Could you check a few things on this model? Use its own coordinates, in mm. A direction names the side the tool comes from. Give positions to 0.01 mm unless a question says otherwise; leave off trailing zeros. Loops run counter-clockwise (first coordinate to the right, second up) from the corner with the lowest first, then second, coordinate; pieces in that order, holes last. Notation, with made-up numbers: M -8,-14.75 L 16,-14.75 A24 cw 16,6.25 Z; hole C -3,65.25 d4. An arc over 180 degrees is marked long. Return JSON: item names as keys, results as strings. Group by question number.
1. Please list where these lines run through material, in increasing order: line 1 (X direction, y = 329.5, z = 139.5); line 2 (Y direction, x = 30, z = -30); line 3 (Y direction, x = 3, z = 236).
2. If we mould it in two halves opening along Z, with no side actions, what happens to faces 1 (the cylindrical face through (-0.85, 342.63, 243.3)), 2 (the flat face through (13.86, 343.08, 242.65)), 3 (the flat face through (19, -3.969, -38)), 4 (the cylindrical face through (-0.98, 739.16, 387.11))? For each: +Z half, -Z half, draft (parallel to the pull), parting line (faces both ways), or undercut.
3. For faces 5 (the flat face through (-0.98, 30.1, -67.07)), 6 (the flat face through (19, -1.984, -38)), 7 (the flat face through (0, 397, 250)), 8 (the cylindrical face through (-0.978, 358.159, 168.827)), which set-ups out of +Z, -Z, +X, -X, +Y, -Y let a thin tool reach every point of the face, with its end or its side?
4. For pin 1 (2 mm diameter, centred on x = -1.5, z = 189, fed in from +Y); pin 2 (1 mm diameter, centred on x = -1, y = 765.5, fed in from -Z); pin 3 (1.6 mm diameter, centred on x = -1, y = 756, fed in from -Z); pin 4 (6.5 mm diameter, centred on y = 340.52, z = 190.1, fed in from -X), each with a flat end and sliding along its axis, tell me the tip position at first contact or that it passes through.
5. If we section it at A-A (y = 702.5): Write out the boundary of the cut face in (x, z).
```python
from build123d import *

# Parameters (mm, degrees)
BASE_FLANGE1_DEPTH                = 1.984375
LOW_RING_SLOT_ONLY_DEPTH          = 915.762916455
HIGH_RING_SLOT_ONLY_DEPTH         = 915.762916455
RING_HOLES_VERTICAL_DEPTH         = 915.762916455
HOOKS_DEPTH                       = 1.984375
CHAIN_PIN_HOLE_D                  = 6.7564
RING_RETAINER_LIP_DEPTH           = 1.984375
ROUNDING_TOP_DEPTH                = 915.762916455
BACK_FLANGE_DEPTH                 = 749.3
BOTTOM_FLANGE_DEPTH               = 76.2
RIVET_HOLES_HOLE_WIZARD_D         = 4.9149
ROUNDING_REMAINING_EDGES_R        = 12.7
BOLT_TO_BASE_HOLE_WIZARD_D        = 6.7564
HOLES_FOR_120LB_CABLE_TIES_D      = 12.7
RIVETS_TO_BACKING_PART_D          = 4.9149
FILLET_FOR_FLANGE_TO_BACK_PIECE_R = 6.35
FILLET_FOR_BOTTOM_FLANGE_R        = 12.7


# Sheet-metal steps are written as plain solids
with BuildPart() as part:
    # Sketch1 → Base-Flange1 (new body)
    with BuildSketch(Plane(origin=(0, 0, 0), x_dir=(0, 0, -1), z_dir=(1, 0, 0))):
        Polygon((-460.1938993, 657.225), (0, 0), (76.2, 0), (76.2, 14.2875), (52.076108029, 14.2875), (-396.113689065, 790.575), (-460.1938993, 790.575), align=None)
    extrude(amount=-BASE_FLANGE1_DEPTH)

    # Sketch2 → low ring slot only (cut, through all)
    with BuildSketch(Plane(origin=(0, 0, 0), x_dir=(0, 0, -1), z_dir=(1, 0, 0))):
        with BuildLine():
            Line((-192.0875, 404.01875), (-188.11875, 404.01875))
            ThreePointArc((-188.11875, 404.01875), (-161.13125, 377.03125), (-188.11875, 350.04375))
            Line((-188.11875, 350.04375), (-192.0875, 350.04375))
            ThreePointArc((-192.0875, 350.04375), (-219.075, 377.03125), (-192.0875, 404.01875))
        make_face()
    extrude(amount=-LOW_RING_SLOT_ONLY_DEPTH, mode=Mode.SUBTRACT)

    # Sketch3 → high ring slot only (cut, through all)
    with BuildSketch(Plane(origin=(0, 0, 0), x_dir=(0, 0, -1), z_dir=(1, 0, 0))):
        with BuildLine():
            Line((-412.75, 785.01875), (-406.4, 785.01875))
            ThreePointArc((-406.4, 785.01875), (-379.4125, 758.03125), (-406.4, 731.04375))
            Line((-406.4, 731.04375), (-412.75, 731.04375))
            ThreePointArc((-412.75, 731.04375), (-439.7375, 758.03125), (-412.75, 785.01875))
        make_face()
    extrude(amount=-HIGH_RING_SLOT_ONLY_DEPTH, mode=Mode.SUBTRACT)

    # Sketch6 → ring holes vertical (cut, through all)
    with BuildSketch(Plane(origin=(0, 0, 0), x_dir=(0, 0, -1), z_dir=(1, 0, 0))):
        Polygon((-157.35409368, 377.03125), (-263.001872817, 560.018571172), (-219.075, 396.08125), (-219.075, 377.03125), (-161.13125, 377.03125), align=None)
        Polygon((-439.7375, 758.03125), (-439.7375, 790.575), (-396.113689065, 790.575), (-377.324546242, 758.03125), (-379.4125, 758.03125), align=None)
    extrude(amount=-RING_HOLES_VERTICAL_DEPTH, mode=Mode.SUBTRACT)

    # Sketch4 → hooks (add)
    with BuildSketch(Plane(origin=(0, 0, 0), x_dir=(0, 0, -1), z_dir=(1, 0, 0))):
        with BuildLine():
            ThreePointArc((54.499076643, 25.965795256), (53.046413321, 20.544381935), (47.625, 21.997045256))
            Line((47.625, 21.997045256), (52.076108029, 14.2875))
            Line((52.076108029, 14.2875), (76.2, 14.2875))
            Line((76.2, 14.2875), (59.4315198, 43.331359673))
            ThreePointArc((59.4315198, 43.331359673), (50.58349781, 45.702180019), (48.212677464, 36.85415803))
            Line((48.212677464, 36.85415803), (54.499076643, 25.965795256))
        make_face()
        with BuildLine():
            ThreePointArc((-97.900923357, 289.93033833), (-99.353586679, 284.508925008), (-104.775, 285.96158833))
            Line((-104.775, 285.96158833), (-85.061678589, 251.817114059))
            ThreePointArc((-85.061678589, 251.817114059), (-88.464633332, 264.517114059), (-85.061678589, 277.217114059))
            Line((-85.061678589, 277.217114059), (-83.998255231, 279.059017344))
            ThreePointArc((-83.998255231, 279.059017344), (-82.296777859, 285.409017344), (-83.998255231, 291.759017344))
            Line((-83.998255231, 291.759017344), (-92.9684802, 307.295902746))
            ThreePointArc((-92.9684802, 307.295902746), (-101.81650219, 309.666723093), (-104.187322536, 300.818701104))
            Line((-104.187322536, 300.818701104), (-97.900923357, 289.93033833))
        make_face()
        with BuildLine():
            ThreePointArc((-264.101571882, 564.122703953), (-264.925165118, 576.688308533), (-260.877417362, 588.612588904))
            Line((-260.877417362, 588.612588904), (-255.028316879, 598.743528119))
            ThreePointArc((-255.028316879, 598.743528119), (-255.028316879, 605.241589069), (-260.655802737, 608.490619543))
            ThreePointArc((-260.655802737, 608.490619543), (-266.499869955, 610.694851427), (-270.7684802, 615.254536332))
            ThreePointArc((-270.7684802, 615.254536332), (-279.61650219, 617.625356679), (-281.987322536, 608.77733469))
            Line((-281.987322536, 608.77733469), (-275.700923357, 597.888971915))
            ThreePointArc((-275.700923357, 597.888971915), (-277.153586679, 592.467558594), (-282.575, 593.920221915))
            Line((-282.575, 593.920221915), (-263.001872817, 560.018571172))
            Line((-263.001872817, 560.018571172), (-264.101571882, 564.122703953))
        make_face()
    extrude(amount=-HOOKS_DEPTH)

    # chain pin hole (through all)
    with Locations(Plane(origin=(0, 0, 0), x_dir=(0, 0, -1), z_dir=(1, 0, 0))):
        with Locations((-260.655802737, 601.992558594)):
            Hole(CHAIN_PIN_HOLE_D / 2)

    # Sketch7 → ring retainer lip (add)
    with BuildSketch(Plane(origin=(0, 0, 0), x_dir=(0, 0, -1), z_dir=(1, 0, 0))):
        with BuildLine():
            Line((-161.13125, 377.03125), (-161.13125, 378.61875))
            ThreePointArc((-161.13125, 378.61875), (-156.36875, 383.38125), (-151.60625, 378.61875))
            Line((-151.60625, 378.61875), (-151.60625, 373.881602199))
            ThreePointArc((-151.60625, 373.881602199), (-150.740765988, 367.307598454), (-148.203295256, 361.181602199))
            Line((-148.203295256, 361.181602199), (-157.35409368, 377.03125))
            Line((-157.35409368, 377.03125), (-161.13125, 377.03125))
        make_face()
        with BuildLine():
            Line((-379.4125, 758.03125), (-379.4125, 759.61875))
            ThreePointArc((-379.4125, 759.61875), (-374.65, 764.38125), (-369.8875, 759.61875))
            Line((-369.8875, 759.61875), (-369.8875, 751.955817539))
            ThreePointArc((-369.8875, 751.955817539), (-369.022015988, 745.381813793), (-366.484545256, 739.255817539))
            Line((-366.484545256, 739.255817539), (-377.324546242, 758.03125))
            Line((-377.324546242, 758.03125), (-379.4125, 758.03125))
        make_face()
    extrude(amount=-RING_RETAINER_LIP_DEPTH)

    # Sketch9 → rounding top (cut, through all)
    with BuildSketch(Plane(origin=(0, 0, 0), x_dir=(0, 0, -1), z_dir=(1, 0, 0))):
        with BuildLine():
            Line((-460.1938993, 790.575), (-460.1938993, 780.34680035))
            ThreePointArc((-460.1938993, 780.34680035), (-457.198128982, 787.579229682), (-449.96569965, 790.575))
            Line((-449.96569965, 790.575), (-460.1938993, 790.575))
        make_face()
        with BuildLine():
            Line((-439.7375, 790.575), (-449.96569965, 790.575))
            ThreePointArc((-449.96569965, 790.575), (-442.733270318, 787.579229682), (-439.7375, 780.34680035))
            Line((-439.7375, 780.34680035), (-439.7375, 790.575))
        make_face()
    extrude(amount=-ROUNDING_TOP_DEPTH, mode=Mode.SUBTRACT)

    # back flange section (across the edge) → back flange (add)
    with BuildSketch(Plane(origin=(0, 645.683578297, 454.534983396), x_dir=(3.4914813388431334e-15, 0.5735764363510447, -0.8191520442889929), z_dir=(0, -0.8191520442889929, -0.5735764363510447))):
        with BuildLine():
            Line((-1.984375, 1.984375), (-1.984375, 25.4))
            Line((-1.984375, 25.4), (0, 25.4))
            Line((0, 25.4), (0, 1.984375))
            ThreePointArc((0, 1.984375), (0.581209981, 0.581209981), (1.984375, 0))
            Line((1.984375, 0), (1.984375, -1.984375))
            ThreePointArc((1.984375, -1.984375), (-0.821955038, -0.821955038), (-1.984375, 1.984375))
        make_face()
    extrude(amount=BACK_FLANGE_DEPTH)

    # bottom flange section (across the edge) → bottom flange (add)
    with BuildSketch(Plane(origin=(0, -1.984375, 0), x_dir=(0, 1, 0), z_dir=(0, 0, -1))):
        with BuildLine():
            Line((-1.984375, 1.984375), (-1.984375, 36.115625))
            Line((-1.984375, 36.115625), (0, 36.115625))
            Line((0, 36.115625), (0, 1.984375))
            ThreePointArc((0, 1.984375), (0.581209981, 0.581209981), (1.984375, 0))
            Line((1.984375, 0), (1.984375, -1.984375))
            ThreePointArc((1.984375, -1.984375), (-0.821955038, -0.821955038), (-1.984375, 1.984375))
        make_face()
    extrude(amount=BOTTOM_FLANGE_DEPTH)

    # rivet holes hole wizard (through all)
    with Locations(Plane(origin=(0, 0, 0), x_dir=(0, 0, -1), z_dir=(1, 0, 0))):
        with Locations((-449.96569965, 734.21875), (-409.575, 721.51875), (-450.6688993, 657.225), (-285.636022628, 580.17206863), (-228.6, 396.08125), (-190.103125, 340.51875), (-107.836022628, 272.213435045), (-9.862916022, 30.692034586), (36.626477372, 21.997045256)):
            Hole(RIVET_HOLES_HOLE_WIZARD_D / 2)

    # rounding remaining edges
    rounding_remaining_edges_edges = [part.edges().sort_by_distance(p)[0] for p in [
        (-0.9921875, 657.225, 460.1938993),
        (-0.9921875, 14.2875, -76.2),
        (-0.9921875, 396.08125, 219.075),
    ]]
    fillet(rounding_remaining_edges_edges, radius=ROUNDING_REMAINING_EDGES_R)

    # bolt to base hole wizard (through all)
    with Locations(Plane(origin=(0, -1.984375, 0), x_dir=(1, 0, 0), z_dir=(0, 1, 0))):
        with Locations((20.240625, 66.675), (20.240625, 9.525)):
            Hole(BOLT_TO_BASE_HOLE_WIZARD_D / 2)

    # holes for 120lb cable ties (through all)
    with Locations(Plane(origin=(0, -1.138190741, 1.625504838), x_dir=(-1, 0, 0), z_dir=(3.580478189914983e-15, 0.5735764363510447, -0.8191520442889927))):
        with Locations((-12.7, 776.923579099), (-12.7, 726.123579099), (-12.7, 446.723579099), (-12.7, 383.223579099)):
            Hole(HOLES_FOR_120LB_CABLE_TIES_D / 2)

    # rivets to backing part (through all)
    with Locations(Plane(origin=(0, -1.138190741, 1.625504838), x_dir=(-1, 0, 0), z_dir=(3.580478189914983e-15, 0.5735764363510447, -0.8191520442889927))):
        with Locations((-12.7, 700.723579099), (-12.7, 491.173579099), (-12.7, 351.473579099), (-12.7, 199.073579099), (-12.7, 59.373579099)):
            Hole(RIVETS_TO_BACKING_PART_D / 2)

    # fillet for flange to back piece
    fillet_for_flange_to_back_piece_edges = [part.edges().sort_by_distance(p)[0] for p in [
        (25.4, 645.114482926, 455.347735815),
        (25.4, 31.32385614, 25.566912057),
    ]]
    fillet(fillet_for_flange_to_back_piece_edges, radius=FILLET_FOR_FLANGE_TO_BACK_PIECE_R)

    # fillet for bottom flange
    fillet_for_bottom_flange_edges = [part.edges().sort_by_distance(p)[0] for p in [
        (36.115625, -2.9765625, 0),
        (36.115625, -2.9765625, -76.2),
    ]]
    fillet(fillet_for_bottom_flange_edges, radius=FILLET_FOR_BOTTOM_FLANGE_R)


solid = part.part
```
Answer:
{
 "1": {"line 1": "x = -1.98 to 0", "line 2": "y = -3.97 to -1.98", "line 3": "y = 330.12 to 333.58"},
 "2": {"face 1": "+Z half", "face 2": "-Z half", "face 3": "draft", "face 4": "undercut"},
 "3": {"face 5": "-Z, +X, -X, +Y", "face 6": "+Z, -Z, +X, +Y", "face 7": "-Z, +X, +Y", "face 8": "+X, -X, +Y"},
 "4": {"pin 1": "stops at y = 350.04", "pin 2": "stops at z = 439.74", "pin 3": "stops at z = 369.89", "pin 4": "stops at x = -1.98"},
 "5": {"outline": "M -1.98,345.26 L 0,345.26 L 0,460.19 L -1.98,460.19 Z"}
}
